from build123d import *

# Parameters (mm, degrees)
DODANIE_WYCI_GNI_CIE1_DEPTH = 1


with BuildPart() as part:
    # Szkic1 → Dodanie-wyciągnięcie1 (new body)
    with BuildSketch(Plane.XY):
        with BuildLine():
            Line((-3.1, -1.267343807), (25.5, -1.267343807))
            Line((25.5, -1.267343807), (25.5, -3.767343807))
            Line((25.5, -3.767343807), (30.1, -3.767343807))
            ThreePointArc((30.1, -3.767343807), (30.382842712, -3.650186519), (30.5, -3.367343807))
            Line((30.5, -3.367343807), (30.5, 11.832656193))
            ThreePointArc((30.5, 11.832656193), (30.382842712, 12.115498905), (30.1, 12.232656193))
            Line((30.1, 12.232656193), (25.5, 12.232656193))
            Line((25.5, 12.232656193), (25.5, 9.732656193))
            Line((25.5, 9.732656193), (-3.1, 9.732656193))
            ThreePointArc((-3.1, 9.732656193), (-3.382842712, 9.615498905), (-3.5, 9.332656193))
            Line((-3.5, 9.332656193), (-3.5, -0.867343807))
            ThreePointArc((-3.5, -0.867343807), (-3.382842712, -1.150186519), (-3.1, -1.267343807))
        make_face()
        with BuildLine():
            Line((18.75, 5.982656193), (20.25, 5.982656193))
            ThreePointArc((20.25, 5.982656193), (22, 4.232656193), (20.25, 2.482656193))
            Line((20.25, 2.482656193), (18.75, 2.482656193))
            ThreePointArc((18.75, 2.482656193), (17, 4.232656193), (18.75, 5.982656193))
        make_face(mode=Mode.SUBTRACT)
        with BuildLine():
            Line((0, 5.982656193), (1.5, 5.982656193))
            ThreePointArc((1.5, 5.982656193), (3.25, 4.232656193), (1.5, 2.482656193))
            Line((1.5, 2.482656193), (0, 2.482656193))
            ThreePointArc((0, 2.482656193), (-1.75, 4.232656193), (0, 5.982656193))
        make_face(mode=Mode.SUBTRACT)
    extrude(amount=DODANIE_WYCI_GNI_CIE1_DEPTH)


solid = part.part
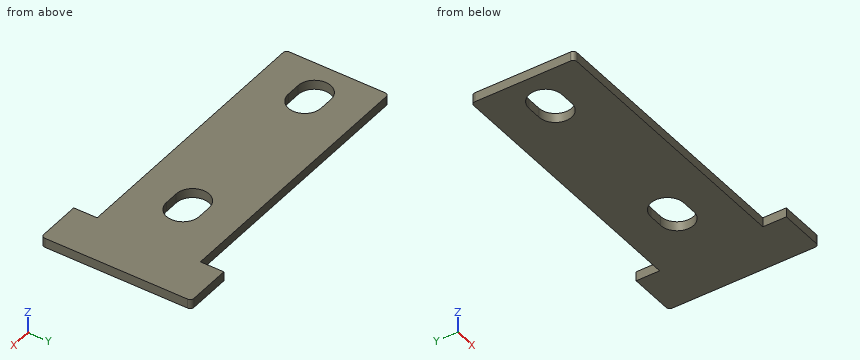
Here's how the part is built. I have some questions about the finished solid (model axes, mm). Round coordinates to 2 decimals unless told otherwise and drop trailing zeros. Loops run counter-clockwise (first coordinate to the right, second up) from the corner with the lowest first, then second, coordinate; pieces in that order, holes last. Notation, with made-up numbers: M 21,45 L 68,45 A37 cw 68,82 Z; hole C 30.25,23 d5. An arc over 180 degrees is marked long. Write each question's results on one line, items separated by ' | '. Start each with the question number.
(1) If I drill on probe 1 along X at (y, z) = (3.5, 0.75); probe 2 along Y at (x, z) = (19, 0.7); probe 3 along Y at (x, z) = (23, 0.2), over which ranges is the centre line in solid material (lowest first)? Write a range as from..to.
(2) I want a section at C-C (y = 5.5). Please give me the cut outline in (x, z), then the cut area to 3 significant figures.
(3) I want a section at A-A (x = 2.5). Please give me the cut outline in (y, z), then the cut area to 3 significant figures.
(4) I want a section at D-D (x = 25). Please give me the cut outline in (y, z).
(5) Will these pins go through, and if not, where does the flat tip stop? P1, Ø0.5, axis at x = 17, z = 0.5, coming from the +Y side; P2, Ø0.5, axis at x = 6.5, z = 0.5, coming from the -Y side.
(6) I want a section at B-B (z = 0.25). Please give me the cut outline in (x, y).
Solved:
1) probe 1: x = -3.5..-1.59, 3.09..17.16, 21.84..30.5 | probe 2: y = -1.27..2.48, 5.98..9.73 | probe 3: y = -1.27..9.73
2) outline: M -3.5,0 L -1.21,0 L -1.21,1 L -3.5,1 Z; M 2.71,0 L 17.54,0 L 17.54,1 L 2.71,1 Z; M 21.46,0 L 30.5,0 L 30.5,1 L 21.46,1 Z | area: 26.2 mm²
3) outline: M -1.27,0 L 2.8,0 L 2.8,1 L -1.27,1 Z; M 5.67,0 L 9.73,0 L 9.73,1 L 5.67,1 Z | area: 8.13 mm²
4) outline: M -1.27,0 L 9.73,0 L 9.73,1 L -1.27,1 Z
5) P1: stops at y = 9.73 | P2: stops at y = -1.27
6) outline: M -3.5,-0.87 A0.4 ccw -3.1,-1.27 L 25.5,-1.27 L 25.5,-3.77 L 30.1,-3.77 A0.4 ccw 30.5,-3.37 L 30.5,11.83 A0.4 ccw 30.1,12.23 L 25.5,12.23 L 25.5,9.73 L -3.1,9.73 A0.4 ccw -3.5,9.33 Z; hole M 0,2.48 L 1.5,2.48 A1.75 ccw 1.5,5.98 L 0,5.98 A1.75 ccw Z; hole M 18.75,2.48 L 20.25,2.48 A1.75 ccw 20.25,5.98 L 18.75,5.98 A1.75 ccw Z
